Check sheet for the modelled part. Datum: model origin and axes. Units: mm. A direction names the side the tool comes from. Give positions to 0.01 mm unless a question says otherwise; leave off trailing zeros. Order: outer loops, then holes, each group sorted by start corner. A loop starts at its lowest first (then second) coordinate and runs counter-clockwise, first axis right, second up.
from build123d import *

# Parameters (mm, degrees)
BOSS_EXTRUDE1_DEPTH = 25
FILLET1_R           = 2


with BuildPart() as part:
    # Sketch1 → Boss-Extrude1 (new body)
    with BuildSketch(Plane.XY):
        with BuildLine():
            Line((-50, 0), (-50, -15))
            Line((-50, -15), (-45, -15))
            Line((-45, -15), (-45, 0))
            ThreePointArc((-45, 0), (0, 45), (45, 0))
            Line((45, 0), (45, -15))
            Line((45, -15), (50, -15))
            Line((50, -15), (50, 0))
            ThreePointArc((50, 0), (0, 50), (-50, 0))
        make_face()
    extrude(amount=BOSS_EXTRUDE1_DEPTH)

    # Fillet1
    fillet1_edges = [part.edges().sort_by_distance(p)[0] for p in [
        (-45, -7.5, 0),
        (-47.5, -15, 0),
        (-50, -7.5, 0),
        (0, 50, 0),
        (-47.5, -15, 25),
        (-45, -7.5, 25),
        (0, 45, 25),
        (45, -7.5, 25),
        (47.5, -15, 25),
        (50, -7.5, 25),
        (0, 50, 25),
        (50, -7.5, 0),
        (-50, -7.5, 25),
        (47.5, -15, 0),
        (45, -7.5, 0),
        (0, 45, 0),
    ]]
    fillet(fillet1_edges, radius=FILLET1_R)


solid = part.part
1) Section check C-C, the plane x = 0. Record the cut outline in (y, z), then the cut area to 3 significant figures.
Recorded:
outline: (45, 2) arc R2 ccw to (47, 0) - (48, 0) arc R2 ccw to (50, 2) - (50, 23) arc R2 ccw to (48, 25) - (47, 25) arc R2 ccw to (45, 23) - close
area: 122 mm2
2) Draft check along X on faces 4 (the face through (49.43, -7.4, 24.4)), 5 (the face through (45, -7, 12)), 6 (the face through (-48, -15, 12)). Enter one of: +X half, -X half, draft (parallel to the pull), parting line (faces both ways), or undercut.
Recorded:
face 4: +X half
face 5: undercut
face 6: draft
3) Section check A-A, the plane y = -8. Record the cut outline in (x, z), then the cut area to 3 significant figures.
Recorded:
outline: (-50, 2) arc R2 ccw to (-48, 0) - (-47, 0) arc R2 ccw to (-45, 2) - (-45, 23) arc R2 ccw to (-47, 25) - (-48, 25) arc R2 ccw to (-50, 23) - close; (45, 2) arc R2 ccw to (47, 0) - (48, 0) arc R2 ccw to (50, 2) - (50, 23) arc R2 ccw to (48, 25) - (47, 25) arc R2 ccw to (45, 23) - close
area: 243 mm2
4) Section check B-B, the plane z = 5.25. Record the cut outline in (x, y).
Recorded:
outline: (-50, -15) - (-45, -15) - (-45, 0) arc R45 cw to (45, 0) - (45, -15) - (50, -15) - (50, 0) arc R50 ccw to (-50, 0) - close
5) Depth check by flat-ended pin: pin 1 Ø3 at (y, z) = (38, 4) entering from -X; pin 2 Ø1 at (x, z) = (-38, 14.5) entering from +Y; pin 3 Ø5 at (y, z) = (34.5, 18) entering from -X. Enter the tip coordinate at first touch or a pass-through.
Recorded:
pin 1: stops at x = -34.17
pin 2: stops at y = 33.07
pin 3: stops at x = -38.42
6) Set-up check for faces 1 (the face through (-47.46, -14.65, 0.87)), 2 (the face through (-45.57, -7.4, 24.4)), 3 (the face through (45.57, -7.61, 0.6)): record each of +Z, -Z, +X, -X, +Y, -Y from which the full face is reachable in a straight line by a thin tool's end or side.
Recorded:
face 1: -Z, +X, -X, -Y
face 2: +Z, -Y
face 3: -Z, -Y
7) Material ranges on L1, parallel to X at y = -7.5, z = 15; L2, parallel to X at y = 5.5, z = 20; L3, parallel to Z at x = 33.5, y = 34.5, recorded low to high.
Recorded:
L1: x = -50 to -45, 45 to 50
L2: x = -49.7 to -44.66, 44.66 to 49.7
L3: z = 0 to 25
